Can you work these out from the model? Positions are in its coordinate system, mm. Round coordinates to 2 decimals unless told otherwise and drop trailing zeros. Write each loop counter-clockwise with the first axis right and the second up, starting at its lowest first coordinate (ties: lowest second). Pieces come first, ordered by that corner, then holes. Notation, with made-up numbers: M -29,20 L 23,20 A32 cw 23,46 Z; hole C 9.5,55.5 d6. An arc over 180 degrees is marked long. Answer as a JSON object with one key per item and string values. Group by question number.
1) Please list where these lines run through material, in increasing order: L1, parallel to Y at x = 187.5, z = 2.55; L2, parallel to X at y = 47.5, z = 3.15; L3, parallel to X at y = 23, z = 1.85. Write a range as [from, to].
2) I'm going to push a flat-ended pin straight in: pin 1 Ø4 at (x, y) = (175, 23) entering from +Z. Where does the tip first touch, or does it pass through?
3) Suppose I cut it at A-A, the plane x = 175. Write out the boundary of the cut face in (y, z), and give its area (3 significant figures).
4) If we mould it in two halves opening along X, with no side actions, what happens to faces 1 (the cylindrical face through (13.962, 21.004, 1.366)), 2 (the flat face through (93.7, 25.4, 0)), 3 (the flat face through (0, 25, 2))? For each: +X half, -X half, draft (parallel to the pull), parting line (faces both ways), or undercut.
5) Suppose I cut it at B-B, the plane y = 23. Write out the boundary of the cut face in (x, z), and give its area (3 significant figures).
from build123d import *

# Parameters (mm, degrees)
ESBO_O1_W                            = 190
ESBO_O1_H                            = 50
RESSALTO_EXTRUS_O1_DEPTH             = 5
FURO_DE_DI_METRO_1_0_1_1_D           = 1
ESCAREADO_PARA_SFHCS_M41_D           = 4.5
ESCAREADO_PARA_SFHCS_M41_CSINK_D     = 8.96
ESCAREADO_PARA_SFHCS_M41_CSINK_ANGLE = 90
ESCAREADO_PARA_SFHCS_M42_D           = 4.5
ESCAREADO_PARA_SFHCS_M42_CSINK_D     = 8.96
ESCAREADO_PARA_SFHCS_M42_CSINK_ANGLE = 90


with BuildPart() as part:
    # Esboço1 → Ressalto-extrusão1 (new body)
    with BuildSketch(Plane.XY):
        with Locations((95, 25)):
            Rectangle(ESBO_O1_W, ESBO_O1_H)
    extrude(amount=RESSALTO_EXTRUS_O1_DEPTH)

    # Furo de diâmetro Ø1.0 (1)1 (through all)
    with Locations(Plane(origin=(2.5, 47.5, 5), x_dir=(1, 0, 0), z_dir=(0, 0, 1))):
        with Locations((0, 0), (0, -45), (185, -45), (185, 0)):
            Hole(FURO_DE_DI_METRO_1_0_1_1_D / 2)

    # Escareado para SFHCS M41 (through all)
    with Locations(Plane(origin=(15, 23, 5), x_dir=(1, 0, 0), z_dir=(0, 0, 1))):
        with Locations((0, 0), (80, 0)):
            CounterSinkHole(ESCAREADO_PARA_SFHCS_M41_D / 2, ESCAREADO_PARA_SFHCS_M41_CSINK_D / 2, counter_sink_angle=ESCAREADO_PARA_SFHCS_M41_CSINK_ANGLE)

    # Escareado para SFHCS M42 (through all)
    with Locations(Plane(origin=(175, 23, 5), x_dir=(1, 0, 0), z_dir=(0, 0, 1))):
        with Locations((0, 0)):
            CounterSinkHole(ESCAREADO_PARA_SFHCS_M42_D / 2, ESCAREADO_PARA_SFHCS_M42_CSINK_D / 2, counter_sink_angle=ESCAREADO_PARA_SFHCS_M42_CSINK_ANGLE)


solid = part.part
Results:
{
 "1": {"L1": "[0, 2], [3, 47], [48, 50]", "L2": "[0, 2], [3, 187], [188, 190]", "L3": "[0, 12.75], [17.25, 92.75], [97.25, 172.75], [177.25, 190]"},
 "2": {"pin 1": "through"},
 "3": {"outline": "M 0,0 L 20.75,0 L 20.75,2.77 L 18.52,5 L 0,5 Z; M 25.25,0 L 50,0 L 50,5 L 27.48,5 L 25.25,2.77 Z", "area": "223 mm^2"},
 "4": {"face 1": "undercut", "face 2": "draft", "face 3": "-X half"},
 "5": {"outline": "M 0,0 L 12.75,0 L 12.75,2.77 L 10.52,5 L 0,5 Z; M 17.25,0 L 92.75,0 L 92.75,2.77 L 90.52,5 L 19.48,5 L 17.25,2.77 Z; M 97.25,0 L 172.75,0 L 172.75,2.77 L 170.52,5 L 99.48,5 L 97.25,2.77 Z; M 177.25,0 L 190,0 L 190,5 L 179.48,5 L 177.25,2.77 Z", "area": "868 mm^2"}
}
